Here's how the part is built. I have some questions about the finished solid (model axes, mm). A direction names the side the tool comes from. Give positions to 0.01 mm unless a question says otherwise; leave off trailing zeros. Loops run counter-clockwise (first coordinate to the right, second up) from the corner with the lowest first, then second, coordinate; pieces in that order, holes last.
Q1. If we section it at B-B (z = 22): Please give me the cut outline in (x, y).
Q2. I need wall thicknesses on line 1 (Z direction, x = -10, y = 14.25); line 2 (Z direction, x = -13.75, y = 12.75); line 3 (X direction, y = 14.5, z = 9.5). Which ranges of each line are inside material? Lowest first, please.
Q3. For faces 1 (the face through (-13, 14, 30)), 2 (the face through (-10, 14, 10)), 3 (the face through (-11.594, 14, 25)), 4 (the face through (-14.176, 13.204, -1.479)), which set-ups out of +Z, -Z, +X, -X, +Y, -Y let a thin tool reach every point of the face, with its end or its side?
Q4. Will these pins go through, and if not, where does the flat tip stop? P1, Ø2, axis at x = -11, z = 24, coming from the -Y side; P2, Ø5, axis at x = -8.5, z = 6.5, coming from the +Y side; P3, Ø3.5, axis at y = 13.5, z = 26.5, coming from the +X side.
Q5. If we section it at A-A (x = -13): Please give me the cut outline in (y, z).
Q6. If we section it at D-D (y = 17.5): Please give me the cut outline in (x, z), plus the area to 3 significant figures.
Q7. If we section it at C-C (y = 13.5): Please give me the cut outline in (x, z).
from build123d import *

# Parameters (mm, degrees)
SKETCH1_R           = 5
BOSS_EXTRUDE1_DEPTH = 10
SKETCH2_R           = 1.707
BOSS_EXTRUDE3_DEPTH = 10
BOSS_EXTRUDE4_DEPTH = 10
SKETCH5_R           = 1.875
BOSS_EXTRUDE5_DEPTH = 3


with BuildPart() as part:
    # Sketch1 → Boss-Extrude1 (new body)
    with BuildSketch(Plane.XY):
        with Locations((-12.444444444, 13.922222222)):
            Circle(SKETCH1_R)
    extrude(amount=BOSS_EXTRUDE1_DEPTH)

    # Sketch2 → Boss-Extrude3 (add)
    with BuildSketch(Plane.XY.offset(10)):
        with Locations((-12.444444444, 13.922222222)):
            Circle(SKETCH2_R)
    extrude(amount=BOSS_EXTRUDE3_DEPTH)

    # Sketch4 → Boss-Extrude4 (add)
    with BuildSketch(Plane.XY.offset(20)):
        with BuildLine():
            Line((-11.593886392, 15.402222222), (-11.593886392, 12.442222222))
            ThreePointArc((-11.593886392, 12.442222222), (-14.151444444, 13.922222222), (-11.593886392, 15.402222222))
        make_face()
    extrude(amount=BOSS_EXTRUDE4_DEPTH)

    # Sketch5 → Boss-Extrude5 (add)
    with BuildSketch(Plane(origin=(0, 0, 0), x_dir=(-1, 0, 0), z_dir=(0, 0, -1))):
        with Locations((12.444444444, 13.922222222)):
            Circle(SKETCH5_R)
    extrude(amount=BOSS_EXTRUDE5_DEPTH)


solid = part.part
Check sheet entries:
1. outline: (-11.59, 12.44) - (-11.59, 15.4) arc R1.71 ccw (long way) to start
2. line 1: z = 0 to 10
2. line 2: z = -3 to 10
2. line 3: x = -17.41 to -7.48
3. face 1: +Z, +X, -X, +Y, -Y
3. face 2: +Z
3. face 3: +Z, +X, +Y, -Y
3. face 4: -Z
4. P1: stops at y = 12.27
4. P2: stops at y = 18.71
4. P3: stops at x = -11.59
5. outline: (8.95, 0) - (12.13, 0) - (12.13, -3) - (15.71, -3) - (15.71, 0) - (18.89, 0) - (18.89, 10) - (15.54, 10) - (15.54, 30) - (12.31, 30) - (12.31, 10) - (8.95, 10) - close
6. outline: (-15.94, 0) - (-8.95, 0) - (-8.95, 10) - (-15.94, 10) - close
6. area: 69.9 mm2
7. outline: (-17.43, 0) - (-14.27, 0) - (-14.27, -3) - (-10.62, -3) - (-10.62, 0) - (-7.46, 0) - (-7.46, 10) - (-10.79, 10) - (-10.79, 20) - (-11.59, 20) - (-11.59, 30) - (-14.1, 30) - (-14.1, 10) - (-17.43, 10) - close
